The listing builds one solid part. Answer for the finished solid, in the listing's coordinates (mm). A direction names the side the tool comes from. Round coordinates to 2 decimals unless told otherwise and drop trailing zeros. Write each loop counter-clockwise with the first axis right and the second up, starting at its lowest first coordinate (ties: lowest second). Pieces come first, ordered by that corner, then holes. Notation, with made-up numbers: M -26,-20.5 L 16,-20.5 A10 cw 16,-8.5 Z; hole C 21,55.5 d4. An arc over 180 degrees is marked long. Put each result on its own line as item: value. Start each with the question number.
```python
from build123d import *

# Parameters (mm, degrees)
SKETCH1_R    = 31.75
BASE_DEPTH   = 1.5875
TRENCH_DEPTH = 31.75


with BuildPart() as part:
    # Sketch1 → Base (new body, symmetric)
    with BuildSketch(Plane.XY):
        Circle(SKETCH1_R)
    extrude(amount=BASE_DEPTH, both=True)

    # Sketch5 → Trench (cut, symmetric)
    with BuildSketch(Plane(origin=(0, 0, 0), x_dir=(0, 0, -1), z_dir=(1, 0, 0))):
        with BuildLine():
            Line((0, -19.05), (1.5875, -19.05))
            ThreePointArc((1.5875, -19.05), (0.397561674, -9.558016141), (0, -8.92e-07))
            Line((0, -8.92e-07), (0, -19.05))
        make_face()
        with BuildLine():
            ThreePointArc((0, -8.92e-07), (0.3975616, 9.558015252), (1.5875, 19.05))
            Line((1.5875, 19.05), (0, 19.05))
            Line((0, 19.05), (0, -8.92e-07))
        make_face()
        with BuildLine():
            Line((1.5875, 19.05), (1.5875, -19.05))
            ThreePointArc((1.5875, -19.05), (0, 0), (1.5875, 19.05))
        make_face()
    extrude(amount=TRENCH_DEPTH, both=True, mode=Mode.SUBTRACT)


solid = part.part
```
Item 1: Section C-C (y = 0) is taken. Give the vertices of the cut face in (x, z).
Item 2: Section D-D (x = -14) is taken. Give the vertices of the cut face in (y, z).
Item 3: Section B-B (z = -1.1) is taken. Give the vertices of the cut face in (x, y), and give its area (3 significant figures).
Item 4: Determine the mould class of faces 3 (the flat face through (0, -24, -1.588)), 4 (the flat face through (0, 0, 0)), 5 (the cylindrical face through (-31.72, 1.4, 0.38)) for opening direction Y: released by +Y, released by -Y, zero draft, split by the parting line, or undercut.
Item 5: Flat-ended cylindrical pins translate along their axes: pin 1 (19 mm diameter, centred on x = 8, y = -1.5, fed in from -Z); pin 2 (0.5 mm diameter, centred on x = 12, z = -0.5, fed in from +Y); pin 3 (1.3 mm diameter, centred on x = 9, z = -1, fed in from -Y). Find the tip coordinate at first contact, or state that the pin passes through.
Item 6: Which of the six approach directions +Z, -Z, +X, -X, +Y, -Y give full straight-line access (tool end or side, diameter ignored) to faces 1 (the flat face through (0, -19.05, -1)), 2 (the flat face through (0, 24, -1.588))?
Item 7: Section A-A (x = 0) is taken. Give the vertices of the cut face in (y, z), and give its area (3 significant figures).
Item 8: Consider line 1 along Z through (x, y) = (19, 9); line 2 along Y through (x, z) = (19.5, -0.75); line 3 along Y through (x, z) = (24, -1.25). Determine where each line is inside the solid, lowest interval first. Write a range as [from, to].
Output values:
1. outline: M -31.75,0 L 31.75,0 L 31.75,1.59 L -31.75,1.59 Z
2. outline: M -28.5,-1.59 L -19.05,-1.59 L -19.05,0 L 19.05,0 L 19.05,-1.59 L 28.5,-1.59 L 28.5,1.59 L -28.5,1.59 Z
3. outline: M -25.4,-19.05 A31.75 ccw 25.4,-19.05 Z; M -25.4,19.05 L 25.4,19.05 A31.75 ccw Z
3. area: 902 mm^2
4. face 3: zero draft
4. face 4: undercut
4. face 5: split by the parting line
5. pin 1: stops at z = 0
5. pin 2: stops at y = 29.5
5. pin 3: stops at y = -30.63
6. face 1: -Z, +X, -X
6. face 2: -Z, +X, -X, +Y, -Y
7. outline: M -31.75,-1.59 L -19.05,-1.59 L -19.05,0 L 19.05,0 L 19.05,-1.59 L 31.75,-1.59 L 31.75,1.59 L -31.75,1.59 Z
7. area: 141 mm^2
8. line 1: z = [0, 1.59]
8. line 2: y = [-25.06, -19.05], [19.05, 25.06]
8. line 3: y = [-20.79, -19.05], [19.05, 20.79]
